from build123d import *

# Parameters (mm, degrees)
BASEHEAD_DEPTH = 5.675
SKETCH4_W      = 0.6
SKETCH4_H      = 11.005553499


# Read off the part's stored shape, not the designer's step: HeadChamfer
with BuildPart() as part:
    # Sketch1 → BaseHead (new body)
    with BuildSketch(Plane(origin=(0, 0, 0), x_dir=(0, 0, -1), z_dir=(1, 0, 0))):
        Polygon((6.5, 3.75277675), (6.5, -3.75277675), (0, -7.505553499), (-6.5, -3.75277675), (-6.5, 3.75277675), (0, 7.505553499), align=None)
    extrude(amount=BASEHEAD_DEPTH)

    # HeadChamfer outline → HeadChamfer (revolve, cut)
    with BuildSketch(Plane.YX):
        Polygon((7.505553503, 0.580556586), (6.499999425, -3.32e-07), (7.505553503, -1.347e-06), align=None)
    revolve(axis=Axis((0, 0, 0), (1, 0, 0)), mode=Mode.SUBTRACT)

    # HeadChamfer 2 outline → HeadChamfer 2 (revolve)
    with BuildSketch(Plane.YX):
        Polygon((4, 5.675), (4, 74.9845), (3.3095, 75.675), (0, 75.675), (0, 5.675), align=None)
    revolve(axis=Axis((0, 0, 0), (1, 0, 0)))

    # Sketch4 → BearingFace (revolve, cut)
    with BuildSketch(Plane.XY, mode=Mode.PRIVATE) as bearingface_sk:
        with Locations((5.375, 12.00277675)):
            Rectangle(SKETCH4_W, SKETCH4_H)
    revolve(bearingface_sk.sketch.rotate(Axis((0, 0, 0), (1, 0, 0)), 90), axis=Axis((0, 0, 0), (1, 0, 0)), mode=Mode.SUBTRACT)


solid = part.part
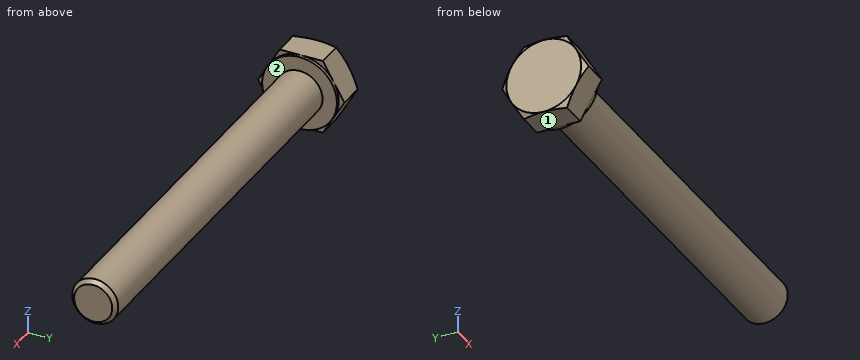
Check sheet for the modelled part. Datum: model origin and axes. Units: mm. Face numbers are marked on the shaded views. A direction names the side the tool comes from. Round coordinates to 2 decimals unless told otherwise and drop trailing zeros. Order: outer loops, then holes, each group sorted by start corner. A loop starts at its lowest first (then second) coordinate and runs counter-clockwise, first axis right, second up.
Q1. Set-up check for the marked faces 1 and 2: record each of +Z, -Z, +X, -X, +Y, -Y from which the full face is reachable in a straight line by a thin tool's end or side.
Filled sheet:
face 1: -Z, +X, -X, +Y, -Y
face 2: +X
Q2. Cross-section at A-A, the plane x = 23. Enter the section's corners in (y, z), plus the area to 3 significant figures.
Filled sheet:
outline: circle Ø8 at (0, 0)
area: 50.3 mm2
Q3. Scan lines: L1, parallel to X at y = 6, z = 2 (3 decimals); L2, parallel to Y at x = 25.5, z = -0.25; L3, parallel to Y at x = 5.5, z = 3.5. Record each from-to range of solid material in increasing order.
Filled sheet:
L1: x = 0 to 5.675
L2: y = -3.99 to 3.99
L3: y = -5.48 to 5.48
Q4. Depth check by flat-ended pin: P1, Ø0.6, axis at y = 7, z = 0, coming from the +X side (3 decimals); P2, Ø3.5, axis at y = 2.5, z = 5, coming from the +X side; P3, Ø2, axis at x = 45.5, z = 0.5, coming from the +Y side. Enter the tip coordinate at first touch or a pass-through.
Filled sheet:
P1: stops at x = 5.075
P2: stops at x = 75.14
P3: stops at y = 4
